Study the drawing (mm; zero at the part's minimum x, y, z) and answer. Give positions to 0.01 mm unless a question says otherwise; leave off trailing zeros. Write each loop counter-clockwise with the first axis right and the second up, starting at its lowest first coordinate (ties: lowest second). Pieces come first, ordered by that corner, then holes. Notation, with made-up numbers: (-31, 30.5) -> (-22, 30.5) arc R29 ccw to (-22, 64.5) -> close; hole circle Ø2 at (-6.75, -18). An arc over 180 degrees is marked (long way). Put each result on its own line as item: value. Start each with the question number.
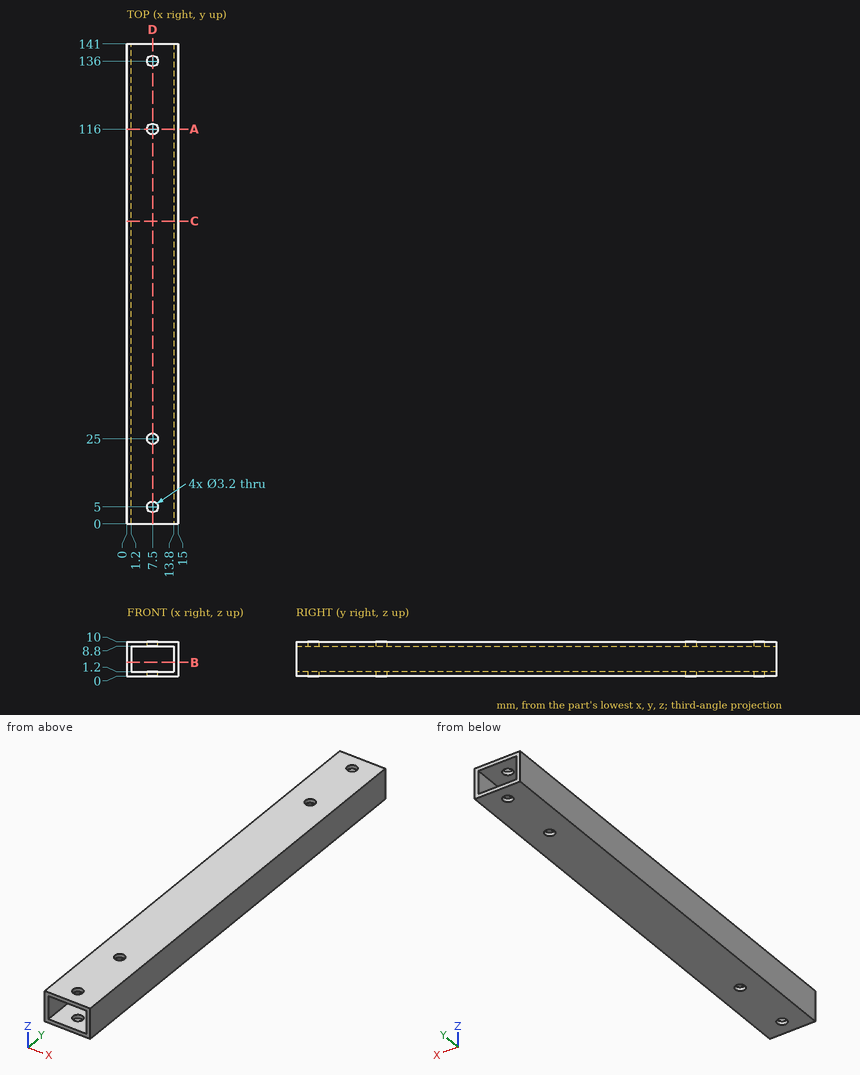
1) A cutting plane is placed at A-A on y = 116. Give the vertices of the cut face in (x, z).
2) A cutting plane is placed at D-D on x = 7.5. State how many separate pieces and enclosed holes the cut face has, and give its area (3 significant figures).
3) Straight lines are drawn through the part: line 1 (Y direction, x = 7.5, z = 9.75); line 2 (X direction, y = 136, z = 0.25); line 3 (Z direction, x = 10, y = 123). For each, find the intervals that lie inside material, in ascending order. Write a range as [from, to].
4) A cutting plane is placed at B-B on z = 4. Give the vertices of the cut face in (x, y).
5) A cutting plane is placed at C-C on y = 89. Give the vertices of the cut face in (x, z), and give its area (3 significant figures).
Results found:
1. outline: (0, 0) -> (5.9, 0) -> (5.9, 1.2) -> (1.2, 1.2) -> (1.2, 8.8) -> (5.9, 8.8) -> (5.9, 10) -> (0, 10) -> close; (9.1, 0) -> (15, 0) -> (15, 10) -> (9.1, 10) -> (9.1, 8.8) -> (13.8, 8.8) -> (13.8, 1.2) -> (9.1, 1.2) -> close
2. separate pieces: 10
2. enclosed holes: 0
2. area: 308 mm²
3. line 1: y = [0, 3.4], [6.6, 23.4], [26.6, 114.4], [117.6, 134.4], [137.6, 141]
3. line 2: x = [0, 5.9], [9.1, 15]
3. line 3: z = [0, 1.2], [8.8, 10]
4. outline: (0, 0) -> (1.2, 0) -> (1.2, 141) -> (0, 141) -> close; (13.8, 0) -> (15, 0) -> (15, 141) -> (13.8, 141) -> close
5. outline: (0, 0) -> (15, 0) -> (15, 10) -> (0, 10) -> close; hole (1.2, 1.2) -> (13.8, 1.2) -> (13.8, 8.8) -> (1.2, 8.8) -> close
5. area: 54.2 mm²
